Verification items for the finished model (mm, model axes). A direction names the side the tool comes from. Round coordinates to 2 decimals unless told otherwise and drop trailing zeros. Write each loop counter-clockwise with the first axis right and the second up, starting at its lowest first coordinate (ties: lowest second). Pieces come first, ordered by that corner, then holes. Notation, with made-up numbers: M 41.5,-7 L 98.5,-7 A29 cw 98.5,13 Z; hole C 46,11.25 d8. An arc over 180 degrees is marked long. One line per question, with ' | ' between items. Start each with the question number.
Q1. Thickness scan on line 1 along X through (y, z) = (-44.5, 7.5); line 2 along X through (y, z) = (-45.5, 13.5); line 3 along Y through (x, z) = (42, 6). Record the ranges inside material, lowest first. Write a range as from..to.
Q2. Cross-section at B-B (y = 0). Record the boundary of the cut face in (x, z), then the cut area to 3 significant figures.
Q3. Release check for a two-part mould opening along Y. For faces 4 (the face through (0.118, 55.343, 9.86)), 5 (the face through (-5, -22, 20)) record: released by +Y, released by -Y, zero draft, split by the parting line, or undercut.
Q4. Cross-section at A-A (x = 50). Record the boundary of the cut face in (y, z).
Q5. Cross-section at D-D (z = 15). Record the boundary of the cut face in (x, y).
Q6. Tool access check on faces 1 (the face through (59.867, -36.893, 9.86)), 2 (the face through (-5, -22, -20)), 3 (the face through (0.118, 55.343, -9.86)). Record the directions out of +Z, -Z, +X, -X, +Y, -Y that give a thin tool (end or side, any length) a straight path to the whole face; none if there is none.
Q7. Cross-section at C-C (z = -13). Record the boundary of the cut face in (x, y), then the cut area to 3 significant figures.
Q8. Gauge pin test, flat ends, axial feed: pin 1 (1 mm diameter, centred on x = 2, z = 0.5, fed in from -Y); pin 2 (4 mm diameter, centred on y = -40.5, z = -15, fed in from -X); pin 3 (10 mm diameter, centred on x = -45, z = 12.5, fed in from -Y). Record the tip position at first contact, or that the pin passes through.
from build123d import *

# Parameters (mm, degrees)
SKETCH1_R                     = 10
BOSS_EXTRUDE1_DEPTH           = 20
BOSS_EXTRUDE1_DRAFT           = 2
BOSS_EXTRUDE1_OTHER_WAY_DEPTH = 20
BOSS_EXTRUDE1_OTHER_WAY_DRAFT = -2


with BuildPart() as part:
    # Sketch1 → Boss-Extrude1 (with draft: the straight prism first)
    with BuildSketch(Plane.XY):
        with BuildLine():
            Line((-12, 50), (-24.079653875, 6.72088307))
            ThreePointArc((-24.079653875, 6.72088307), (-24.928097247, 1.894721), (-24.81883517, -3.004233816))
            ThreePointArc((-24.81883517, -3.004233816), (-30.762049538, -19.776348187), (-47.717387131, -25.174694658))
            ThreePointArc((-47.717387131, -25.174694658), (-61.713032142, -49.370425713), (-35.03522611, -41.027395935))
            ThreePointArc((-35.03522611, -41.027395935), (-26.046643252, -25.670606045), (-8.378996809, -23.554031767))
            ThreePointArc((-8.378996809, -23.554031767), (0, -25), (8.378996809, -23.554031767))
            ThreePointArc((8.378996809, -23.554031767), (26.046643252, -25.670606045), (35.03522611, -41.027395935))
            ThreePointArc((35.03522611, -41.027395935), (61.713032142, -49.370425713), (47.717387131, -25.174694658))
            ThreePointArc((47.717387131, -25.174694658), (30.762049538, -19.776348187), (24.81883517, -3.004233816))
            ThreePointArc((24.81883517, -3.004233816), (24.928097247, 1.894721), (24.079653875, 6.72088307))
            Line((24.079653875, 6.72088307), (12, 50))
            ThreePointArc((12, 50), (0, 62), (-12, 50))
        make_face()
        with Locations((50, -40)):
            Circle(SKETCH1_R, mode=Mode.SUBTRACT)
        with Locations((-50, -40)):
            Circle(SKETCH1_R, mode=Mode.SUBTRACT)
        with BuildLine():
            ThreePointArc((5, 50), (0, 55), (-5, 50))
            Line((-5, 50), (-19.048602886, 6.095139711))
            ThreePointArc((-19.048602886, 6.095139711), (0, -20), (19.048602886, 6.095139711))
            Line((19.048602886, 6.095139711), (5, 50))
        make_face(mode=Mode.SUBTRACT)
    extrude(amount=BOSS_EXTRUDE1_DEPTH)
    # Boss-Extrude1: the draft: its side faces are tilted about the plane it starts from
    boss_extrude1_sides = [part.faces().sort_by_distance(p)[0] for p in [
        (24.928097247, 1.894721, 10),
        (18.039826938, 28.360441535, 10),
        (0, 62, 10),
        (-18.039826938, 28.360441535, 10),
        (-24.928097247, 1.894721, 10),
        (-30.762049538, -19.776348187, 10),
        (-61.713032142, -49.370425713, 10),
        (-26.046643252, -25.670606045, 10),
        (0, -25, 10),
        (26.046643252, -25.670606045, 10),
        (61.713032142, -49.370425713, 10),
        (30.762049538, -19.776348187, 10),
        (40, -40, 10),
        (-60, -40, 10),
        (0, -20, 10),
        (-12.024301443, 28.047569856, 10),
        (0, 55, 10),
        (12.024301443, 28.047569856, 10),
    ]]
    draft(boss_extrude1_sides, Plane.XY, BOSS_EXTRUDE1_DRAFT)


with BuildPart() as boss_extrude1_other_way_tool:
    # Sketch1 → Boss-Extrude1 other way (with draft: the straight prism first)
    with BuildSketch(Plane.XY):
        with BuildLine():
            Line((-12, 50), (-24.079653875, 6.72088307))
            ThreePointArc((-24.079653875, 6.72088307), (-24.928097247, 1.894721), (-24.81883517, -3.004233816))
            ThreePointArc((-24.81883517, -3.004233816), (-30.762049538, -19.776348187), (-47.717387131, -25.174694658))
            ThreePointArc((-47.717387131, -25.174694658), (-61.713032142, -49.370425713), (-35.03522611, -41.027395935))
            ThreePointArc((-35.03522611, -41.027395935), (-26.046643252, -25.670606045), (-8.378996809, -23.554031767))
            ThreePointArc((-8.378996809, -23.554031767), (0, -25), (8.378996809, -23.554031767))
            ThreePointArc((8.378996809, -23.554031767), (26.046643252, -25.670606045), (35.03522611, -41.027395935))
            ThreePointArc((35.03522611, -41.027395935), (61.713032142, -49.370425713), (47.717387131, -25.174694658))
            ThreePointArc((47.717387131, -25.174694658), (30.762049538, -19.776348187), (24.81883517, -3.004233816))
            ThreePointArc((24.81883517, -3.004233816), (24.928097247, 1.894721), (24.079653875, 6.72088307))
            Line((24.079653875, 6.72088307), (12, 50))
            ThreePointArc((12, 50), (0, 62), (-12, 50))
        make_face()
        with Locations((50, -40)):
            Circle(SKETCH1_R, mode=Mode.SUBTRACT)
        with Locations((-50, -40)):
            Circle(SKETCH1_R, mode=Mode.SUBTRACT)
        with BuildLine():
            ThreePointArc((5, 50), (0, 55), (-5, 50))
            Line((-5, 50), (-19.048602886, 6.095139711))
            ThreePointArc((-19.048602886, 6.095139711), (0, -20), (19.048602886, 6.095139711))
            Line((19.048602886, 6.095139711), (5, 50))
        make_face(mode=Mode.SUBTRACT)
    extrude(amount=-BOSS_EXTRUDE1_OTHER_WAY_DEPTH)
    # Boss-Extrude1 other way: the draft: its side faces are tilted about the plane it starts from
    boss_extrude1_other_way_sides = [boss_extrude1_other_way_tool.faces().sort_by_distance(p)[0] for p in [
        (24.928097247, 1.894721, -10),
        (18.039826938, 28.360441535, -10),
        (0, 62, -10),
        (-18.039826938, 28.360441535, -10),
        (-24.928097247, 1.894721, -10),
        (-30.762049538, -19.776348187, -10),
        (-61.713032142, -49.370425713, -10),
        (-26.046643252, -25.670606045, -10),
        (0, -25, -10),
        (26.046643252, -25.670606045, -10),
        (61.713032142, -49.370425713, -10),
        (30.762049538, -19.776348187, -10),
        (40, -40, -10),
        (-60, -40, -10),
        (0, -20, -10),
        (-12.024301443, 28.047569856, -10),
        (0, 55, -10),
        (12.024301443, 28.047569856, -10),
    ]]
    draft(boss_extrude1_other_way_sides, Plane.XY, BOSS_EXTRUDE1_OTHER_WAY_DRAFT)


with BuildPart() as part_1:
    add(part.part)

    # Boss-Extrude1 other way: add boss_extrude1_other_way_tool
    add(boss_extrude1_other_way_tool.part)


solid = part_1.part
Determined:
1) line 1: x = -64.03..-59.22, -40.78..-35.97, 35.97..40.78, 59.22..64.03 | line 2: x = -63.45..-58.91, -41.09..-36.55, 36.55..41.09, 58.91..63.45 | line 3: y = -52.44..-46.34, -33.66..-25.44
2) outline: M -25,0 L -24.3,-20 L -20.7,-20 L -20,0 L -20.7,20 L -24.3,20 Z; M 20,0 L 20.7,-20 L 24.3,-20 L 25,0 L 24.3,20 L 20.7,20 Z | area: 344 mm²
3) face 4: undercut | face 5: zero draft
4) outline: M -55,0 L -54.3,-20 L -50.7,-20 L -50,0 L -50.7,20 L -54.3,20 Z; M -30,0 L -29.3,-20 L -25.7,-20 L -25,0 L -25.7,20 L -29.3,20 Z
5) outline: M -47.8,-25.69 A14.48 ccw long -35.56,-40.99 A20.52 cw -8.2,-23.06 A24.48 ccw 8.2,-23.06 A20.52 cw 35.56,-40.99 A14.48 ccw long 47.8,-25.69 A20.52 cw 24.3,-2.94 A24.48 ccw 23.58,6.58 L 11.48,49.93 A11.48 ccw long -11.48,49.93 L -23.58,6.58 A24.48 ccw -24.3,-2.94 A20.52 cw Z; hole C -50,-40 d21.05; hole M -19.55,6.25 A20.52 ccw long 19.55,6.25 L 5.52,50.08 A5.52 ccw -5.52,50.08 Z; hole C 50,-40 d21.05
6) face 1: +Z | face 2: -Z, +X, -X, +Y, -Y | face 3: -Z
7) outline: M -47.79,-25.62 A14.55 ccw long -35.49,-41 A20.45 cw -8.23,-23.13 A24.55 ccw 8.23,-23.13 A20.45 cw 35.49,-41 A14.55 ccw long 47.79,-25.62 A20.45 cw 24.37,-2.95 A24.55 ccw 23.64,6.6 L 11.55,49.94 A11.55 ccw long -11.55,49.94 L -23.64,6.6 A24.55 ccw -24.37,-2.95 A20.45 cw Z; hole C -50,-40 d20.91; hole M -19.48,6.23 A20.45 ccw long 19.48,6.23 L 5.45,50.07 A5.45 ccw -5.45,50.07 Z; hole C 50,-40 d20.91 | area: 2,110 mm²
8) pin 1: stops at y = -24.94 | pin 2: stops at x = -64.54 | pin 3: stops at y = -54.64
